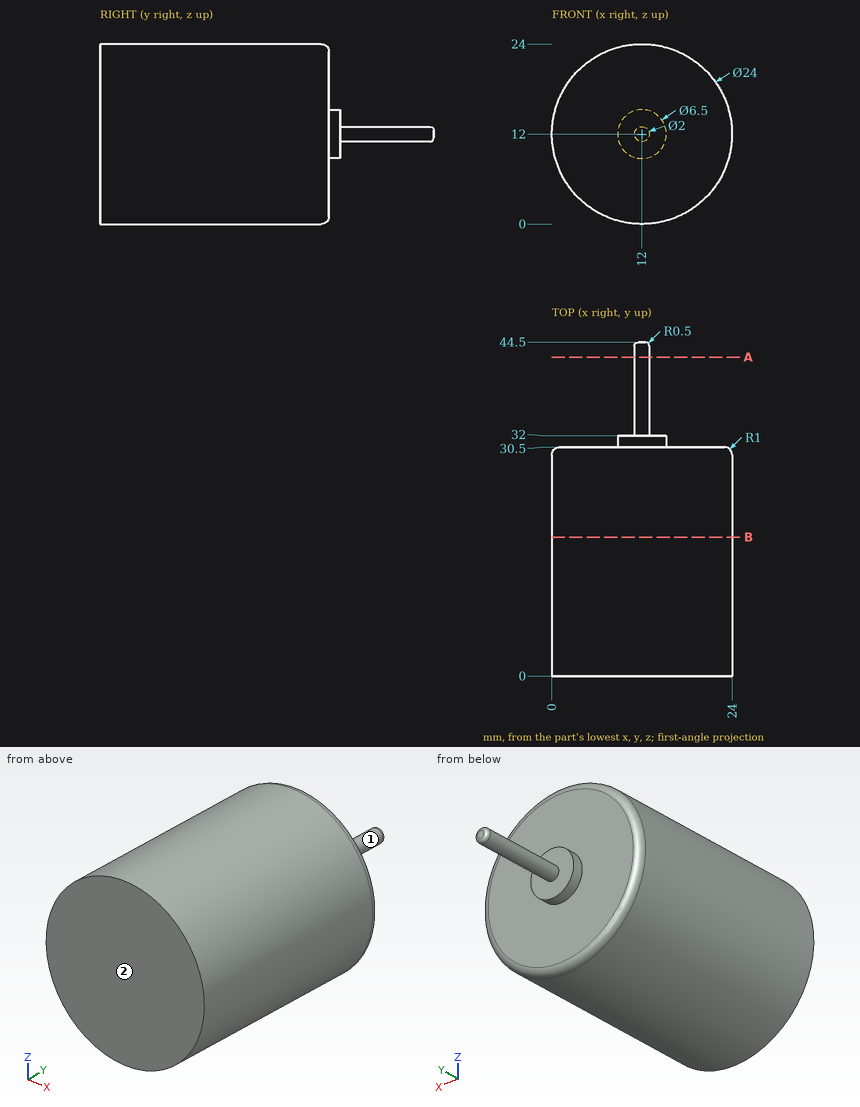
For this review, use the dimensioned drawing (mm, ordinates from the lowest corner) and the shaded views. A direction names the side the tool comes from. Round coordinates to 2 decimals unless told otherwise and drop trailing zeros. Write each loop counter-clockwise with the first axis right and the second up, starting at its lowest first coordinate (ties: lowest second). Pieces come first, ordered by that corner, then holes. Notation, with made-up numbers: M -21,29 L 29,29 A22 ccw 29,42 Z; hole C -33.5,49.5 d4. An arc over 180 degrees is marked long. Answer as CSV lines item,"result". Start each with the question number.
Q1. Clearance check with flat-ended pins moving along their axes: P1, Ø6.5, axis at x = 15, z = 9.5, coming from the +Y side; P2, Ø3, axis at x = 17, z = 18, coming from the +Y side; P3, Ø4, axis at y = 9.5, z = 6, coming from the -X side. State where each tip first meets the part, or that it passes through.
Q2. Wall thickness on line 1 along X through (y, z) = (28, 12); line 2 along Y through (x, z) = (8.25, 10.5); line 3 along Y through (x, z) = (9.75, 10.25): over which ranges is each line inside the solid? List them lowest first.
Q3. Tool access review of the marked faces 1 and 2: name each direction out of +Z, -Z, +X, -X, +Y, -Y from which nothing blocks a thin tool from reaching the whole face with its end or side.
Q4. Consider section A-A, the plane y = 42.5. Give the boundary of the cut face in (x, z).
Q5. Consider section B-B, the plane y = 18.5. Give the boundary of the cut face in (x, z).
Result set:
1,P1,"stops at y = 44.48"
1,P2,"stops at y = 30.5"
1,P3,"stops at x = 0.69"
2,line 1,"x = 0 to 24"
2,line 2,"y = 0 to 30.5"
2,line 3,"y = 0 to 32"
3,face 1,"+Y"
3,face 2,"+Z, -Z, +X, -X, -Y"
4,outline,"C 12,12 d2"
5,outline,"C 12,12 d24"
